The model under review builds one solid part; all positions refer to its coordinate system, in mm. Coordinates: 2 decimals unless noted, no trailing zeros. Order: outer loops, then holes, each group sorted by start corner. A loop starts at its lowest first (then second) coordinate and runs counter-clockwise, first axis right, second up. Notation, with made-up numbers: (-0.5, -12) -> (21.5, -12) arc R28 ccw to (21.5, 23) -> close; hole circle Ø8 at (9, -31). An arc over 180 degrees is marked (long way). Put each result on its own line as item: value.
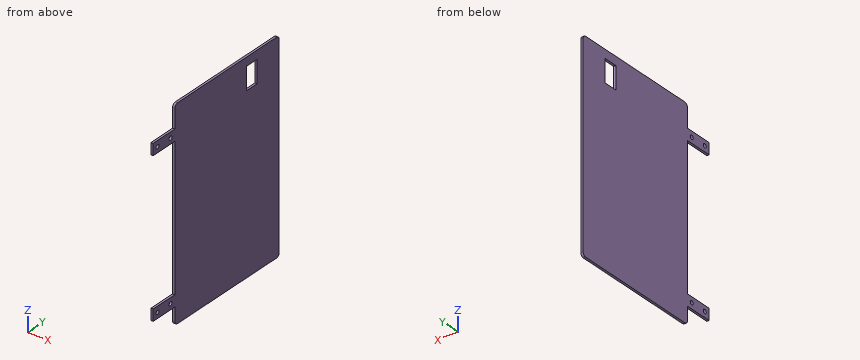
from build123d import *

# Parameters (mm, degrees)
SKETCH2_W             = 360
SKETCH2_H             = 240
BOSS_EXTRUDE2_DEPTH   = 2
FILLET1_R             = 6
SKETCH3_W             = 40
SKETCH3_H             = 25
CUT_EXTRUDE1_DEPTH    = 237.921928069
SKETCH4_W             = 20
SKETCH4_H             = 50
BOSS_EXTRUDE3_DEPTH   = 2
M8X1_0_TAPPED_HOLE1_D = 7


with BuildPart() as part:
    # Sketch2 → Boss-Extrude2 (new, symmetric)
    with BuildSketch(Plane(origin=(0, 0, 0), x_dir=(0, 0, -1), z_dir=(1, 0, 0))):
        with Locations((0, -34)):
            Rectangle(SKETCH2_W, SKETCH2_H)
    extrude(amount=BOSS_EXTRUDE2_DEPTH, both=True)

    # Fillet1
    fillet1_edges = [part.edges().sort_by_distance(p)[0] for p in [
        (0, -154, -180),
        (0, -154, 180),
        (0, 86, 180),
        (0, 86, -180),
    ]]
    fillet(fillet1_edges, radius=FILLET1_R)

    # Sketch3 → Cut-Extrude1 (cut, through all)
    with BuildSketch(Plane(origin=(2, 0, 0), x_dir=(0, 0, -1), z_dir=(1, 0, 0))):
        with Locations((-145, 23)):
            Rectangle(SKETCH3_W, SKETCH3_H)
    extrude(amount=-CUT_EXTRUDE1_DEPTH, mode=Mode.SUBTRACT)

    # Sketch4 → Boss-Extrude3 (add, symmetric)
    with BuildSketch(Plane(origin=(0, 0, 0), x_dir=(0, 0, -1), z_dir=(1, 0, 0))):
        with Locations((-130, -179)):
            Rectangle(SKETCH4_W, SKETCH4_H)
        with Locations((140.074687189, -179)):
            Rectangle(SKETCH4_W, SKETCH4_H)
    extrude(amount=BOSS_EXTRUDE3_DEPTH, both=True)

    # M8x1.0 Tapped Hole1 (through all)
    with Locations(Plane(origin=(2, 0, 0), x_dir=(0, 0, -1), z_dir=(1, 0, 0))):
        with Locations((-129.925312811, -194), (-129.925312811, -164), (140.074687189, -194), (140.074687189, -164)):
            Hole(M8X1_0_TAPPED_HOLE1_D / 2)


solid = part.part
Item 1: For line 1 (Z direction, x = 1.1, y = -164); line 2 (Z direction, x = 1.75, y = 32); line 3 (Y direction, x = -0.8, z = 84.5), list the stretches that pass through material, from the lowest coordinate up. Write a range as from..to.
Answers below:
line 1: -150.07..-143.57, -136.57..-130.07, 120..126.43, 133.43..140
line 2: -180..125, 165..180
line 3: -154..86
Item 2: Consider section C-C on z = -75. Write out the cut boundary in (x, y).
Answers below:
outline: (-2, -154) -> (2, -154) -> (2, 86) -> (-2, 86) -> close
Item 3: For pin 1 Ø5.5 at (y, z) = (-194, -140.07) entering from -X; pin 2 Ø2 at (x, z) = (-0.5, 29.5) entering from -Y; pin 3 Ø1.2 at (x, y) = (0, -171) entering from -Z, all flat-tipped, find the tip position at first contact; note any pin that passes through.
Answers below:
pin 1: through
pin 2: y = -154
pin 3: z = -150.07
Item 4: Consider section B-B on x = -1.3. Write out the cut boundary in (y, z).
Answers below:
outline: (-204, -150.07) -> (-154, -150.07) -> (-154, -174) arc R6 ccw to (-148, -180) -> (80, -180) arc R6 ccw to (86, -174) -> (86, 174) arc R6 ccw to (80, 180) -> (-148, 180) arc R6 ccw to (-154, 174) -> (-154, 140) -> (-204, 140) -> (-204, 120) -> (-154, 120) -> (-154, -130.07) -> (-204, -130.07) -> close; hole circle Ø7 at (-194, -140.07); hole circle Ø7 at (-194, 129.93); hole circle Ø7 at (-164, -140.07); hole circle Ø7 at (-164, 129.93); hole (10.5, 125) -> (35.5, 125) -> (35.5, 165) -> (10.5, 165) -> close
Item 5: Consider section A-A on y = 30.5. Write out the cut boundary in (x, z), and give its area (3 significant figures).
Answers below:
outline: (-2, -180) -> (2, -180) -> (2, 125) -> (-2, 125) -> close; (-2, 165) -> (2, 165) -> (2, 180) -> (-2, 180) -> close
area: 1,280 mm^2
